Could you check a few things on this model? Use its own coordinates, in mm. A direction names the side the tool comes from. Give positions to 0.01 mm unless a question says otherwise; leave off trailing zeros. Order: outer loops, then holes, each group sorted by start corner. A loop starts at its lowest first (then second) coordinate and runs counter-clockwise, first axis right, second up. Notation, with made-up numbers: (56, 61) -> (68, 61) arc R3 cw to (68, 65) -> close; hole circle Ø4 at (6, 40). An arc over 180 degrees is marked (long way). Write each question's results on one line, items separated by ' | '.
```python
from build123d import *

# Parameters (mm, degrees)
SKETCH1_W           = 20
SKETCH1_H           = 14
BOSS_EXTRUDE1_DEPTH = 2
CHAMFER3_SIZE       = 2
SKETCH2_W           = 14
SKETCH2_H           = 8
BOSS_EXTRUDE2_DEPTH = 3
CUT_EXTRUDE1_DEPTH  = 16.165750888
SKETCH5_W           = 16
SKETCH5_H           = 10
BOSS_EXTRUDE3_DEPTH = 4
SKETCH6_R           = 2.017871448
SKETCH6_R_2         = 1.817871448
SKETCH6_W           = 4.259238865
SKETCH6_H           = 0.3
CUT_EXTRUDE2_DEPTH  = 1.5


with BuildPart() as part:
    # Sketch1 → Boss-Extrude1 (new body)
    with BuildSketch(Plane.XY):
        Rectangle(SKETCH1_W, SKETCH1_H)
    extrude(amount=BOSS_EXTRUDE1_DEPTH)

    # Chamfer3
    chamfer3_edges = [part.edges().sort_by_distance(p)[0] for p in [
        (-10, 0, 0),
        (0, -7, 0),
        (0, 7, 0),
        (10, 0, 0),
    ]]
    chamfer(chamfer3_edges, length=CHAMFER3_SIZE - 0.0001)  # a hair under: the kernel refuses the full size

    # Sketch2 → Boss-Extrude2 (add)
    with BuildSketch(Plane(origin=(0, 0, 0), x_dir=(-1, 0, 0), z_dir=(0, 0, -1))):
        Rectangle(SKETCH2_W, SKETCH2_H)
    extrude(amount=BOSS_EXTRUDE2_DEPTH)

    # Sketch3 → Cut-Extrude1 (cut, through all)
    with BuildSketch(Plane(origin=(0, 4, 0), x_dir=(1, 0, 0), z_dir=(0, 1, 0))):
        with BuildLine():
            add(Edge.make_bspline(
                [(6.607979195, 3), (-0.019315958, 0.580486074), (-7, 0)],
                knots=[0, 0, 0, 1, 1, 1], degree=2))
            Line((6.607979195, 3), (-7, 3))
            Line((-7, 3), (-7, 0))
        make_face()
        Polygon((6.607979195, 3), (7, 0), (7, 3), align=None)
    extrude(amount=-CUT_EXTRUDE1_DEPTH, mode=Mode.SUBTRACT)

    # Sketch5 → Boss-Extrude3 (add)
    with BuildSketch(Plane.XY.offset(2)):
        Rectangle(SKETCH5_W, SKETCH5_H)
    extrude(amount=BOSS_EXTRUDE3_DEPTH)

    # Sketch6 → Cut-Extrude2 (cut)
    # profile 1 of 2: a face of its own
    with BuildSketch(Plane(origin=(6.607979195, -4, -3), x_dir=(-0.9915700128560622, 0, 0.12957202477629515), z_dir=(-0.12957202477629515, 0, -0.9915700128560622))):
        with Locations((3.092933481, 4)):
            Circle(SKETCH6_R)
        with Locations((3.092933481, 4)):
            Circle(SKETCH6_R_2, mode=Mode.SUBTRACT)
    # profile 2 of 2: a face of its own
    with BuildSketch(Plane(origin=(6.607979195, -4, -3), x_dir=(-0.9915700128560622, 0, 0.12957202477629515), z_dir=(-0.12957202477629515, 0, -0.9915700128560622))):
        with Locations((10.0255244, 4)):
            Rectangle(SKETCH6_W, SKETCH6_H)
    extrude(amount=-CUT_EXTRUDE2_DEPTH, mode=Mode.SUBTRACT)


solid = part.part
```
Q1. For faces 4 (the flat face through (0, -4.4, 0)), 5 (the flat face through (8, 0, 4)), 6 (the flat face through (3, 4, -1)), which set-ups out of +Z, -Z, +X, -X, +Y, -Y let a thin tool reach every point of the face, with its end or its side?
Here are the results:
face 4: -Z | face 5: +Z, +X, +Y, -Y | face 6: -Z, +X, -X, +Y
Q2. I need wall thicknesses on line 1 along Y through (x, z) = (-0.5, 3); line 2 along X through (y, z) = (-2, 5.5); line 3 along Y through (x, z) = (4.5, -2). Which ranges of each line are inside material? Lowest first, please.
Here are the results:
line 1: y = -5 to 5 | line 2: x = -8 to 8 | line 3: y = -4 to -1.82, -1.59 to 1.59, 1.82 to 4
Q3. Thinking about a two-plate mould opening in Y: for faces 1 (the cylindrical face through (5.473, 0.08, -1.83)), 2 (the flat face through (3, -4, -1)), 3 (the flat face through (0, 5, 4)), which applies, +Y half, -Y half, draft (parallel to the pull), parting line (faces both ways), or undercut?
Here are the results:
face 1: undercut | face 2: -Y half | face 3: +Y half
Q4. I'm going to push flat-ended pins straight in: pin 1 Ø3 at (y, z) = (2.5, 2.5) entering from +X; pin 2 Ø4 at (x, y) = (-2.5, -4) entering from -Z; pin 3 Ø5 at (x, z) = (6, 1.5) entering from +Y. Where does each tip first touch, or does it pass through?
Here are the results:
pin 1: stops at x = 10 | pin 2: stops at z = -0.96 | pin 3: stops at y = 7
Q5. Suppose I cut it at B-B on z = 3. Please give me the cut outline in (x, y), and give its area (3 significant figures).
Here are the results:
outline: (-8, -5) -> (8, -5) -> (8, 5) -> (-8, 5) -> close | area: 160 mm²
